Source: CAD feature listing. Evaluate the final solid. Frame: model axes, mm. Face numbers are marked on the shaded views. A direction names the side the tool comes from. Give positions to 0.01 mm unless a question says otherwise; leave off trailing zeros. Loops run counter-clockwise (first coordinate to the right, second up) from the corner with the lowest first, then second, coordinate; pieces in that order, holes last. Notation, with made-up numbers: (49.25, 15.5) -> (74.25, 15.5) arc R12 ccw to (74.25, 32.5) -> close; hole circle Ø8 at (87.5, -22.5). An arc over 180 degrees is marked (long way). Put each result on its own line as item: value.
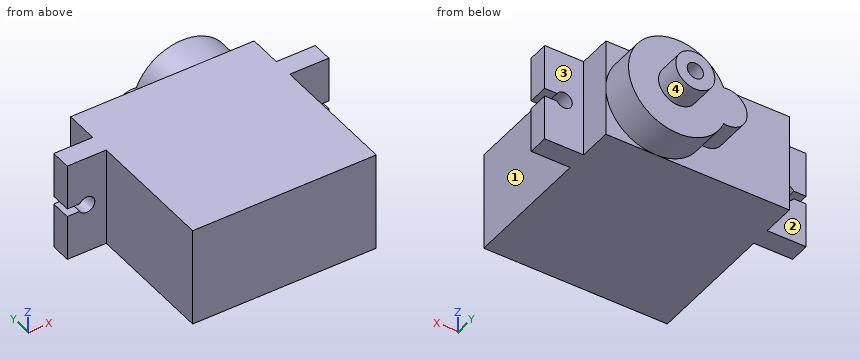
```python
from build123d import *

# Parameters (mm, degrees)
SKETCH1_W           = 22.6
SKETCH1_H           = 12.2
BOSS_EXTRUDE1_DEPTH = 22.6
SKETCH4_W           = 12.2
SKETCH4_H           = 2.5
BOSS_EXTRUDE2_DEPTH = 4.8
SKETCH5_W           = 12.2
SKETCH5_H           = 2.5
BOSS_EXTRUDE3_DEPTH = 4.8
BOSS_EXTRUDE4_DEPTH = 4.2
SKETCH9_R           = 2.4
BOSS_EXTRUDE5_DEPTH = 3.2
SKETCH10_R          = 1
CUT_EXTRUDE1_DEPTH  = 3.2
CUT_EXTRUDE2_DEPTH  = 26.271921177
CUT_EXTRUDE3_DEPTH  = 26.271921177


with BuildPart() as part:
    # Sketch1 → Boss-Extrude1 (new body)
    with BuildSketch(Plane(origin=(0, 0, 0), x_dir=(1, 0, 0), z_dir=(0, 1, 0))):
        Rectangle(SKETCH1_W, SKETCH1_H)
    extrude(amount=BOSS_EXTRUDE1_DEPTH)

    # Sketch4 → Boss-Extrude2 (add)
    with BuildSketch(Plane.ZY.offset(11.3)):
        with Locations((0, 17.25)):
            Rectangle(SKETCH4_W, SKETCH4_H)
    extrude(amount=BOSS_EXTRUDE2_DEPTH)

    # Sketch5 → Boss-Extrude3 (add)
    with BuildSketch(Plane(origin=(11.3, 0, 0), x_dir=(0, 0, -1), z_dir=(1, 0, 0))):
        with Locations((0, 17.25)):
            Rectangle(SKETCH5_W, SKETCH5_H)
    extrude(amount=BOSS_EXTRUDE3_DEPTH)

    # Sketch8 → Boss-Extrude4 (add)
    with BuildSketch(Plane(origin=(0, 22.6, 0), x_dir=(1, 0, 0), z_dir=(0, 1, 0))):
        with BuildLine():
            ThreePointArc((-0.427868852, -2.353102671), (11.3, 0), (-0.427868852, 2.353102671))
            ThreePointArc((-0.427868852, 2.353102671), (-3.3, 0), (-0.427868852, -2.353102671))
        make_face()
    extrude(amount=BOSS_EXTRUDE4_DEPTH)

    # Sketch9 → Boss-Extrude5 (add)
    with BuildSketch(Plane(origin=(0, 26.8, 0), x_dir=(1, 0, 0), z_dir=(0, 1, 0))):
        with Locations(Location((5.2, 0, 0), (0, 0, 270))):
            Circle(SKETCH9_R)
    extrude(amount=BOSS_EXTRUDE5_DEPTH)

    # Sketch10 → Cut-Extrude1 (cut)
    with BuildSketch(Plane(origin=(0, 30, 0), x_dir=(1, 0, 0), z_dir=(0, 1, 0))):
        with Locations(Location((5.2, 0, 0), (0, 0, 270))):
            Circle(SKETCH10_R)
    extrude(amount=-CUT_EXTRUDE1_DEPTH, mode=Mode.SUBTRACT)

    # Sketch12 → Cut-Extrude2 (cut, through all)
    with BuildSketch(Plane(origin=(0, 18.5, 0), x_dir=(1, 0, 0), z_dir=(0, 1, 0))):
        with BuildLine():
            Line((16.1, 0.5), (16.1, -0.5))
            Line((16.1, -0.5), (14.566025404, -0.5))
            ThreePointArc((14.566025404, -0.5), (12.7, 0), (14.566025404, 0.5))
            Line((14.566025404, 0.5), (16.1, 0.5))
        make_face()
    extrude(amount=-CUT_EXTRUDE2_DEPTH, mode=Mode.SUBTRACT)

    # Sketch13 → Cut-Extrude3 (cut, through all)
    with BuildSketch(Plane(origin=(0, 18.5, 0), x_dir=(1, 0, 0), z_dir=(0, 1, 0))):
        with BuildLine():
            Line((-16.1, 0.5), (-16.1, -0.5))
            Line((-16.1, -0.5), (-14.566025404, -0.5))
            ThreePointArc((-14.566025404, -0.5), (-12.7, 0), (-14.566025404, 0.5))
            Line((-14.566025404, 0.5), (-16.1, 0.5))
        make_face()
    extrude(amount=-CUT_EXTRUDE3_DEPTH, mode=Mode.SUBTRACT)


solid = part.part
```
(1) Line query: probe 1 along Z at (x, y) = (-13.7, 17.05); probe 2 along Y at (x, z) = (-8, 4); probe 3 along X at (y, z) = (5.25, -4.25). Output: solid intervals per line, ascending. Write a range as from..to.
Calculated:
probe 1: z = -6.1..-1, 1..6.1
probe 2: y = 0..22.6
probe 3: x = -11.3..11.3
(2) First-contact query: P1, Ø4, axis at x = -14, z = 3, coming from the +Y side; P2, Ø5.5, axis at x = 14, z = -0.5, coming from the +Y side; P3, Ø4, axis at y = 9.5, z = -1.5, coming from the +X side. Flat tips, straight axial feed; report the tip coordinate or a pass-through.
Calculated:
P1: stops at y = 18.5
P2: stops at y = 26.8
P3: stops at x = 11.3
(3) Section B-B on x = -0.9. Return loops of the section in (y, z).
Calculated:
outline: (0, -6.1) -> (22.6, -6.1) -> (22.6, -2.4) -> (26.8, -2.4) -> (26.8, 2.4) -> (22.6, 2.4) -> (22.6, 6.1) -> (0, 6.1) -> close
(4) Section D-D on z = -5.5. Return loops of the section in (x, y), then the cut area to 3 significant figures.
Calculated:
outline: (-16.1, 16) -> (-11.3, 16) -> (-11.3, 0) -> (11.3, 0) -> (11.3, 16) -> (16.1, 16) -> (16.1, 18.5) -> (11.3, 18.5) -> (11.3, 22.6) -> (7.84, 22.6) -> (7.84, 26.8) -> (2.56, 26.8) -> (2.56, 22.6) -> (-11.3, 22.6) -> (-11.3, 18.5) -> (-16.1, 18.5) -> close
area: 557 mm²
(5) Section C-C on y = 16.5. Return loops of the section in (x, z), then the cut area to 3 significant figures.
Calculated:
outline: (-16.1, -6.1) -> (16.1, -6.1) -> (16.1, -0.5) -> (14.57, -0.5) arc R1 cw (long way) to (14.57, 0.5) -> (16.1, 0.5) -> (16.1, 6.1) -> (-16.1, 6.1) -> (-16.1, 0.5) -> (-14.57, 0.5) arc R1 cw (long way) to (-14.57, -0.5) -> (-16.1, -0.5) -> close
area: 384 mm²
(6) Section A-A on x = 13.7. Return loops of the section in (y, z), then the cut area to 3 significant figures.
Calculated:
outline: (16, -6.1) -> (18.5, -6.1) -> (18.5, -1) -> (16, -1) -> close; (16, 1) -> (18.5, 1) -> (18.5, 6.1) -> (16, 6.1) -> close
area: 25.5 mm²
(7) Reachability of the marked faces 1, 2, 3 and 4 from +Z, -Z, +X, -X, +Y, -Y: full face, straight path, thin tool, end or side. Return the list, or none.
Calculated:
face 1: +Z, -Z, +X, -Y
face 2: +Z, -Z, -X, +Y
face 3: +Z, -Z, +X, +Y
face 4: +Y
